Solid Edge part; units mm, degrees
sketch "Sketch1" plane through (0, 0, 0) normal (0, 0, 1) x (1, 0, 0)
  line L0 (-18.5425, 0) -> (17.4575, 0)
  line L1 (17.4575, 0) -> (17.4575, 36)
  line L2 (17.4575, 36) -> (-18.5425, 36)
  line L3 (-18.5425, 36) -> (-18.5425, 0)
extrude "Protrusion1" add sketch "Sketch1" along normal blind 34
sketch "Sketch2" plane through (-0.5425, 18, 34) normal (0, 0, 1) x (1, 0, 0)
  line L0 (-16, -16) -> (16, -16)
  line L1 (16, -16) -> (16, 16)
  line L2 (16, 16) -> (-16, 16)
  line L3 (-16, 16) -> (-16, -16)
extrude "ExtrudedCutout_1" cut sketch "Sketch2" against normal blind 32
sketch "Sketch3" plane through (-18.5425, 18, 17) normal (-1, 0, 0) x (0, -1, 0)
  line L0 (-18, -17) -> (-14, -17)
  line L1 (-14, -17) -> (-14, -13)
  line L2 (-14, -13) -> (-18, -13)
  line L3 (-18, -13) -> (-18, -17)
extrude "ExtrudedProtrusion_2" add sketch "Sketch3" along normal blind 5
sketch "Sketch4" plane through (-18.5425, 18, 17) normal (-1, 0, 0) x (0, -1, 0)
  circle A0 centre (2.3474, -10.3644) radius 1
extrude "ExtrudedProtrusion_3" add sketch "Sketch4" along normal blind 5
For this review, take the finished solid that the model builds, in its own axes (mm). A direction names the side the tool comes from. Coordinates: 2 decimals unless noted, no trailing zeros. Order: outer loops, then holes, each group sorted by start corner. A loop starts at its lowest first (then second) coordinate and runs counter-clockwise, first axis right, second up. Notation, with made-up numbers: (65, 13.5) -> (102, 13.5) arc R30 ccw to (102, 51.5) -> close; hole circle Ø11 at (-8, -30). An arc over 180 degrees is marked (long way). Answer as CSV lines item,"result".
Q1. Draft analysis for pull direction Y (two halves, no side actions). For faces 5 (the face through (0, 34, 18)), 6 (the face through (-23.542, 34, 2)), 7 (the face through (-3, 36, 17)), 8 (the face through (-1, 18, 2)), state which applies: released by +Y, released by -Y, zero draft, split by the parting line, or undercut.
Model answer:
face 5,"undercut"
face 6,"zero draft"
face 7,"released by +Y"
face 8,"undercut"
Q2. We need section B-B (z = 24). State the section outline as (x, y) points, plus the area to 3 significant figures.
Model answer:
outline,"(-18.54, 0) -> (17.46, 0) -> (17.46, 36) -> (-18.54, 36) -> close; hole (-16.54, 2) -> (15.46, 2) -> (15.46, 34) -> (-16.54, 34) -> close"
area,"272 mm2"
Q3. Clearance check with flat-ended pins moving along their axes: pin 1 Ø8 at (y, z) = (28.5, 18) entering from -X; pin 2 Ø16 at (x, y) = (0, 15) entering from +Z; pin 3 Ø12 at (x, z) = (-10, 25) entering from -Y; pin 4 Ø1.2 at (x, z) = (-22, 2.5) entering from -Y. State where each tip first meets the part, or that it passes through.
Model answer:
pin 1,"stops at x = -18.54"
pin 2,"stops at z = 2"
pin 3,"stops at y = 0"
pin 4,"stops at y = 32"
Q4. We need section A-A (y = 3). State the section outline as (x, z) points.
Model answer:
outline,"(-18.54, 0) -> (17.46, 0) -> (17.46, 34) -> (15.46, 34) -> (15.46, 2) -> (-16.54, 2) -> (-16.54, 34) -> (-18.54, 34) -> close"
Q5. We need section C-C (x = 6). State the section outline as (y, z) points.
Model answer:
outline,"(0, 0) -> (36, 0) -> (36, 34) -> (34, 34) -> (34, 2) -> (2, 2) -> (2, 34) -> (0, 34) -> close"
Q6. For faces 1 (the face through (15.458, 18, 18)), 2 (the face through (-21, 34, 4)), 3 (the face through (-21, 32, 2)), 4 (the face through (-21.008, 14.699, 6.335)), list the 3-axis set-ups (+Z, -Z, +X, -X, +Y, -Y) from which the entire face can be reached by the end or side of a thin tool; tool diameter is ignored.
Model answer:
face 1,"+Z"
face 2,"+Z, -X, +Y, -Y"
face 3,"+Z, -Z, -X, -Y"
face 4,"-X"
Q7. Wall thickness on line 1 along X through (y, z) = (20, 12); line 2 along Y through (x, z) = (-14, 4.5); line 3 along Z through (x, y) = (2, 23): over which ranges is each line inside the solid? List them lowest first. Write a range as [from, to].
Model answer:
line 1,"x = [-18.54, -16.54], [15.46, 17.46]"
line 2,"y = [0, 2], [34, 36]"
line 3,"z = [0, 2]"
